from build123d import *

# Parameters (mm, degrees)
SKETCH1_W           = 30
SKETCH1_H           = 3
SKETCH1_W_2         = 3
SKETCH1_H_2         = 22.5
BOSS_EXTRUDE1_DEPTH = 3


with BuildPart() as part:
    # Sketch1 → Boss-Extrude1 (new body)
    with BuildSketch(Plane(origin=(0, 0, 0), x_dir=(0, 0, -1), z_dir=(1, 0, 0))):
        with BuildLine():
            Line((75.25, -13), (93, -13))
            ThreePointArc((93, -13), (96.535533906, -11.535533906), (98, -8))
            Line((98, -8), (98, 88))
            ThreePointArc((98, 88), (96.535533906, 91.535533906), (93, 93))
            Line((93, 93), (-3, 93))
            ThreePointArc((-3, 93), (-6.535533906, 91.535533906), (-8, 88))
            Line((-8, 88), (-8, -8))
            ThreePointArc((-8, -8), (-6.535533906, -11.535533906), (-3, -13))
            Line((-3, -13), (14.75, -13))
            ThreePointArc((14.75, -13), (16.340990258, -12.340990258), (17, -10.75))
            Line((17, -10.75), (17, -10.25))
            ThreePointArc((17, -10.25), (17.659009742, -8.659009742), (19.25, -8))
            Line((19.25, -8), (70.75, -8))
            ThreePointArc((70.75, -8), (72.340990258, -8.659009742), (73, -10.25))
            Line((73, -10.25), (73, -10.75))
            ThreePointArc((73, -10.75), (73.659009742, -12.340990258), (75.25, -13))
        make_face()
        Polygon((0, 0), (0, 19.5), (-3, 19.5), (-3, -3), (0, -3), align=None, mode=Mode.SUBTRACT)
        Polygon((90, 0), (90, 19.5), (93, 19.5), (93, -3), (90, -3), align=None, mode=Mode.SUBTRACT)
        with Locations((45, 85.5)):
            Rectangle(SKETCH1_W, SKETCH1_H, mode=Mode.SUBTRACT)
        with Locations((45, -1.5)):
            Rectangle(SKETCH1_W, SKETCH1_H, mode=Mode.SUBTRACT)
        with Locations((91.5, 53.25)):
            Rectangle(SKETCH1_W_2, SKETCH1_H_2, mode=Mode.SUBTRACT)
        with Locations((-1.5, 53.25)):
            Rectangle(SKETCH1_W_2, SKETCH1_H_2, mode=Mode.SUBTRACT)
    extrude(amount=BOSS_EXTRUDE1_DEPTH)


solid = part.part
Verification items for the finished model (mm, model axes). A direction names the side the tool comes from. Coordinates: 2 decimals unless noted, no trailing zeros. Write each loop counter-clockwise with the first axis right and the second up, starting at its lowest first coordinate (ties: lowest second). Pieces come first, ordered by that corner, then holes. Notation, with made-up numbers: (-9.5, 59) -> (20.5, 59) arc R36 ccw to (20.5, 95) -> close; hole circle Ø9 at (40.25, -23). An arc over 180 degrees is marked (long way). One line per item, written item: value. Start each with the question number.
Q1. Cross-section at B-B on z = -39. Enter the section's corners in (x, y).
Q2. Cross-section at C-C on x = 0.5. State how many separate pieces and enclosed holes the cut face has, and give its area (3 significant figures).
Q3. Access from +Z, -Z, +X, -X, +Y, -Y to the whole of each face (thin tool, end or side, straight path). Record for faces 4 (the flat face through (0, 41, -44)), 5 (the flat face through (1, -3, 2)), 6 (the cylindrical face through (1.48, -8.68, -17.64)).
Q4. Thickness scan on L1, parallel to Z at x = 1.65, y = 17.5; L2, parallel to Y at x = 0.7, z = -51.5; L3, parallel to Y at x = 0.95, z = -20. Record the ranges inside material, lowest first. Write a range as from..to.
Q5. Cross-section at A-A on y = 4. Enter the section's corners in (x, z).
Q6. Mould release check, pull along Z, two halves, no side actions. Record for faces 1 (the cylindrical face through (1, 91, -97)), 2 (the flat face through (1, 93, -46)), 3 (the flat face through (1, 8, -93)): pulls with the +Z half, pulls with the -Z half, needs draft (parallel to the pull), parting line crosses it, or undercut.
Q7. Go/stop test with flat-tipped pins: P1, Ø1, axis at x = 2, z = -38.5, coming from the -Y side; P2, Ø0.6, axis at x = 2, y = -10.5, coming from the +Z side. Record where each tip stops, or that it passes through.
Q8. Cross-section at D-D on z = -24.5. Enter the section's corners in (x, y).
Checked values:
1. outline: (0, -8) -> (3, -8) -> (3, -3) -> (0, -3) -> close; (0, 0) -> (3, 0) -> (3, 84) -> (0, 84) -> close; (0, 87) -> (3, 87) -> (3, 93) -> (0, 93) -> close
2. separate pieces: 1
2. enclosed holes: 6
2. area: 10,500 mm²
3. face 4: +Z, -Z, -X, +Y, -Y
3. face 5: +X, -X
3. face 6: +X, -X, -Y
4. L1: z = -98..-93, -90..0, 3..8
4. L2: y = -8..-3, 0..84, 87..93
4. L3: y = -8..93
5. outline: (0, -98) -> (3, -98) -> (3, -93) -> (0, -93) -> close; (0, -90) -> (3, -90) -> (3, 0) -> (0, 0) -> close; (0, 3) -> (3, 3) -> (3, 8) -> (0, 8) -> close
6. face 1: pulls with the -Z half
6. face 2: needs draft
6. face 3: undercut
7. P1: stops at y = -8
7. P2: stops at z = 7.49
8. outline: (0, -8) -> (3, -8) -> (3, 93) -> (0, 93) -> close
